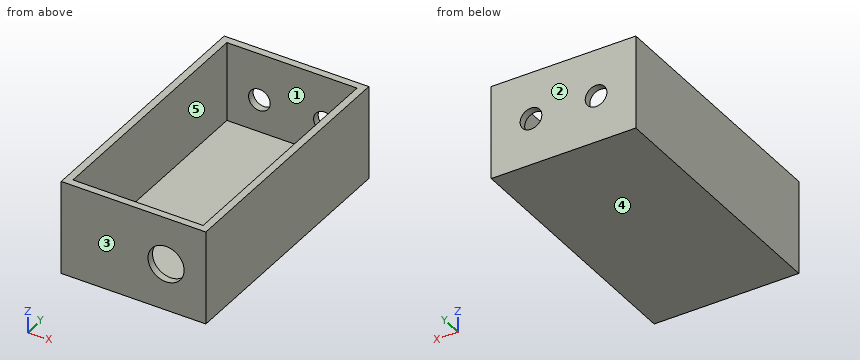
from build123d import *

# Parameters (mm, degrees)
F0_W     = 40
F0_H     = 72
F1_DEPTH = 26
F2_W     = 36
F2_H     = 68
F3_DEPTH = 22
F4_R     = 5
F5_DEPTH = 25
F6_R     = 3
F7_DEPTH = 25


with BuildPart() as f1:
    # F0 (on Top) → F1 (new body)
    with BuildSketch(Plane.XY):
        Rectangle(F0_W, F0_H)
    extrude(amount=F1_DEPTH)

    # F2 (on face) → F3 (cut)
    with BuildSketch(Plane.XY.offset(26)):
        Rectangle(F2_W, F2_H)
    extrude(amount=-F3_DEPTH, mode=Mode.SUBTRACT)

    # F4 (on face) → F5 (cut)
    with BuildSketch(Plane.XZ.offset(36)):
        with Locations((9, 13)):
            Circle(F4_R)
    extrude(amount=-F5_DEPTH, mode=Mode.SUBTRACT)

    # F6 (on face) → F7 (cut)
    with BuildSketch(Plane(origin=(0, 36, 0), x_dir=(-1, 0, 0), z_dir=(0, 1, 0))):
        with Locations((-9, 13)):
            Circle(F6_R)
        with Locations((9, 13)):
            Circle(F6_R)
    extrude(amount=-F7_DEPTH, mode=Mode.SUBTRACT)


solid = f1.part
The model under review builds one solid part; all positions refer to its coordinate system, in mm. Face numbers are marked on the shaded views. A direction names the side the tool comes from. Round coordinates to 2 decimals unless told otherwise and drop trailing zeros. Order: outer loops, then holes, each group sorted by start corner. A loop starts at its lowest first (then second) coordinate and runs counter-clockwise, first axis right, second up. Notation, with made-up numbers: (17.25, 55.25) -> (48.25, 55.25) arc R29 cw to (48.25, 77.25) -> close; hole circle Ø8 at (84, 11.5). An arc over 180 degrees is marked (long way). Write item = value, one per line. Start each with the question number.
Item 1: Consider section B-B on x = -9. Write out the cut boundary in (y, z).
Item 2: Mouldability with a two-part tool opening along Y and no side actions: class the marked faces 1, 2 and 3 as released by +Y, released by -Y, zero draft, split by the parting line, or undercut.
Item 3: Consider section D-D on z = 4.75. Write out the cut boundary in (x, y), plus the area to 3 significant figures.
Item 4: Consider section C-C on x = 9. Write out the cut boundary in (y, z).
Item 5: Consider section A-A on z = 13. Write out the cut boundary in (x, y), plus the area to 3 significant figures.
Item 6: For the marked faces 4 and 5, list the 3-axis set-ups (+Z, -Z, +X, -X, +Y, -Y) from which the entire face can be reached by the end or side of a thin tool; tool diameter is ignored.
Item 7: Clearance check with flat-ended pins moving along their axes: pin 1 Ø5 at (x, y) = (2.5, 0.5) entering from +Z; pin 2 Ø8 at (x, z) = (9, 13) entering from -Y. State where each tip first meets the part, or that it passes through.
Item 8: For line 1 along X through (y, z) = (-9, 8); line 2 along Z through (x, y) = (-9, 34.45); line 3 along Y through (x, z) = (4, 14), list the stretches that pass through material, from the lowest coordinate up.
Conclusion:
q1.outline = (-36, 0) -> (36, 0) -> (36, 10) -> (34, 10) -> (34, 4) -> (-34, 4) -> (-34, 26) -> (-36, 26) -> close; (34, 16) -> (36, 16) -> (36, 26) -> (34, 26) -> close
q2.face_1 = undercut
q2.face_2 = released by +Y
q2.face_3 = released by -Y
q3.outline = (-20, -36) -> (20, -36) -> (20, 36) -> (-20, 36) -> close; hole (-18, -34) -> (18, -34) -> (18, 34) -> (-18, 34) -> close
q3.area = 432 mm2
q4.outline = (-36, 0) -> (36, 0) -> (36, 10) -> (34, 10) -> (34, 4) -> (-34, 4) -> (-34, 8) -> (-36, 8) -> close; (-36, 18) -> (-34, 18) -> (-34, 26) -> (-36, 26) -> close; (34, 16) -> (36, 16) -> (36, 26) -> (34, 26) -> close
q5.outline = (-20, -36) -> (4, -36) -> (4, -34) -> (-18, -34) -> (-18, 34) -> (-12, 34) -> (-12, 36) -> (-20, 36) -> close; (-6, 34) -> (6, 34) -> (6, 36) -> (-6, 36) -> close; (12, 34) -> (18, 34) -> (18, -34) -> (14, -34) -> (14, -36) -> (20, -36) -> (20, 36) -> (12, 36) -> close
q5.area = 388 mm2
q6.face_4 = -Z, +X, -X, +Y, -Y
q6.face_5 = +Z
q7.pin_1 = 4
q7.pin_2 = 34
q8.line_1 = -20 to -18, 18 to 20
q8.line_2 = 0 to 10, 16 to 26
q8.line_3 = -36 to -34, 34 to 36
